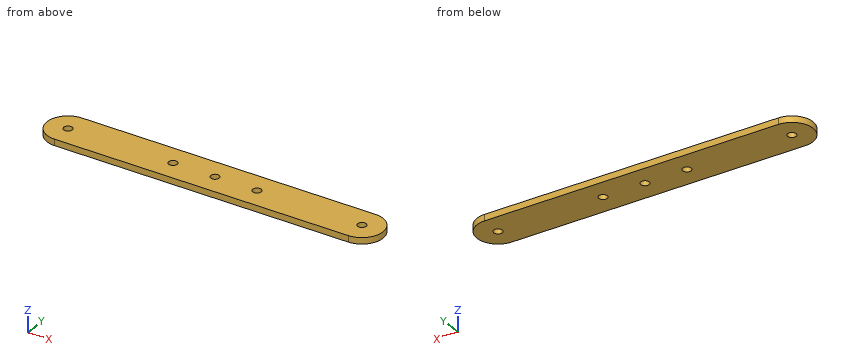
```python
from build123d import *

# Parameters (mm, degrees)
ESQUISSE1_R        = 1
BOSS_EXTRU_2_DEPTH = 1.5


with BuildPart() as part:
    # Esquisse1 → Boss.-Extru.2 (new body)
    with BuildSketch(Plane.XY):
        with BuildLine():
            Line((-35, 5), (35, 5))
            ThreePointArc((35, 5), (40, 0), (35, -5))
            Line((35, -5), (-35, -5))
            ThreePointArc((-35, -5), (-40, 0), (-35, 5))
        make_face()
        with Locations((-35, 0)):
            Circle(ESQUISSE1_R, mode=Mode.SUBTRACT)
        Circle(ESQUISSE1_R, mode=Mode.SUBTRACT)
        with Locations((35, 0)):
            Circle(ESQUISSE1_R, mode=Mode.SUBTRACT)
        with Locations((-10, 0)):
            Circle(ESQUISSE1_R, mode=Mode.SUBTRACT)
        with Locations((10, 0)):
            Circle(ESQUISSE1_R, mode=Mode.SUBTRACT)
    extrude(amount=BOSS_EXTRU_2_DEPTH)


solid = part.part
```
Here's how the part is built. I have some questions about the finished solid (model axes, mm). Round coordinates to 2 decimals unless told otherwise and drop trailing zeros. Order: outer loops, then holes, each group sorted by start corner. A loop starts at its lowest first (then second) coordinate and runs counter-clockwise, first axis right, second up. Notation, with made-up numbers: M -39,-11 L -15,-11 A15 ccw -15,-1 Z; hole C 37,67.5 d2. An arc over 180 degrees is marked long. Answer in a Markdown table with one row per item.
Item 1: If I drill on L1, parallel to Y at x = -10, z = 0.65; L2, parallel to X at y = -0.5, z = 0.1; L3, parallel to X at y = 3.5, z = 0.15, over which ranges is the centre line in solid material (lowest first)? Write a range as from..to.
A:
| item | result |
|---|---|
| L1 | y = -5..-1, 1..5 |
| L2 | x = -39.97..-35.87, -34.13..-10.87, -9.13..-0.87, 0.87..9.13, 10.87..34.13, 35.87..39.97 |
| L3 | x = -38.57..38.57 |
Item 2: Imagine slicing it at A-A, the plane x = -10. Write out the boundary of the cut face in (y, z).
A:
| item | result |
|---|---|
| outline | M -5,0 L -1,0 L -1,1.5 L -5,1.5 Z; M 1,0 L 5,0 L 5,1.5 L 1,1.5 Z |
Item 3: Imagine slicing it at C-C, the plane y = 0. Write out the boundary of the cut face in (x, z), and give its area (3 significant figures).
A:
| item | result |
|---|---|
| outline | M -40,0 L -36,0 L -36,1.5 L -40,1.5 Z; M -34,0 L -11,0 L -11,1.5 L -34,1.5 Z; M -9,0 L -1,0 L -1,1.5 L -9,1.5 Z; M 1,0 L 9,0 L 9,1.5 L 1,1.5 Z; M 11,0 L 34,0 L 34,1.5 L 11,1.5 Z; M 36,0 L 40,0 L 40,1.5 L 36,1.5 Z |
| area | 105 mm2 |
Item 4: Imagine slicing it at B-B, the plane z = 0.3. Write out the boundary of the cut face in (x, y).
A:
| item | result |
|---|---|
| outline | M -35,-5 L 35,-5 A5 ccw 35,5 L -35,5 A5 ccw Z; hole C -35,0 d2; hole C -10,0 d2; hole C 0,0 d2; hole C 10,0 d2; hole C 35,0 d2 |
Item 5: Imagine slicing it at D-D, the plane y = 4.25. Write out the boundary of the cut face in (x, z), and give its area (3 significant figures).
A:
| item | result |
|---|---|
| outline | M -37.63,0 L 37.63,0 L 37.63,1.5 L -37.63,1.5 Z |
| area | 113 mm2 |
